from build123d import *


with BuildPart() as part:
    # Sketch2 → Revolve1 (revolve)
    with BuildSketch(Plane.XY, mode=Mode.PRIVATE) as revolve1_sk:
        with BuildLine():
            Line((-140, 65), (19.954223861, 65))
            add(Edge.make_bspline(
                [(19.954223861, 65), (21.016036949, 65.019364415), (23.155754142, 65.047133931), (27.308551501, 65.056367434), (32.353198871, 64.984650174), (38.152864496, 64.771098732), (45.567688357, 64.32486699), (54.255095035, 63.479775498), (63.813883484, 62.056181028), (72.567017756, 60.273903927), (83.242872896, 57.488773814), (94.867435167, 53.373767517), (106.518267243, 47.87450931), (116.322752818, 42.298539812), (124.736044428, 37.141710874), (132.197152427, 32.876448525), (139.118198638, 29.887038599), (146.009326462, 28.369530473), (153.724403185, 28.498164942), (163.163761497, 30.774524673), (172.93972339, 34.968320575), (182.118464779, 39.947020221), (189.735067248, 44.546297097), (198.139536323, 50.063346613), (205.847141634, 55.467762959), (212.465840749, 60.301248812), (217.661687494, 64.186041861), (222.197887983, 67.650369213), (225.939095655, 70.549100478), (227.873902956, 72.061946017), (228.830902799, 72.813469047)],
                knots=[0.000111982, 0.000111982, 0.000111982, 0.000111982, 0.007923607, 0.015735232, 0.031358482, 0.046981733, 0.062604983, 0.093851484, 0.125097984, 0.156344485, 0.187590985, 0.250083986, 0.312576987, 0.375069989, 0.43756299, 0.500055991, 0.562548992, 0.625041993, 0.687534994, 0.750027995, 0.812520997, 0.843767497, 0.875013998, 0.906260498, 0.937506999, 0.953130249, 0.968753499, 0.98437675, 0.992188375, 1, 1, 1, 1], degree=3))
            Line((228.830902799, 72.813469047), (231.918980433, 68.881068187))
            add(Edge.make_bspline(
                [(20.045394315, 60.000831274), (155.133832213, 62.464455683), (107.158700851, -29.09201306), (231.918980433, 68.881068187)],
                knots=[0.000111982, 0.000111982, 0.000111982, 0.000111982, 1, 1, 1, 1], degree=3))
            ThreePointArc((20.045394315, 60.000831274), (19.999810983, 60.000207823), (19.954223861, 60))
            Line((19.954223861, 60), (-140, 60))
            Line((-140, 60), (-140, 65))
        make_face()
    revolve(revolve1_sk.sketch.rotate(Axis((-140, 0, 0), (1, 0, 0)), 90), axis=Axis((-140, 0, 0), (1, 0, 0)))


solid = part.part
Verification items for the finished model (mm, model axes). Coordinates: 2 decimals unless noted, no trailing zeros. Loops run counter-clockwise (first coordinate to the right, second up) from the corner with the lowest first, then second, coordinate; pieces in that order, holes last. Notation, with made-up numbers: (55.25, 34.25) -> (90.25, 34.25) arc R27 ccw to (90.25, 56.25) -> close; hole circle Ø1 at (89, -18). An arc over 180 degrees is marked (long way). Answer as a JSON object with one key per item and string values. Group by question number.
Item 1: Mould release check, pull along Y, two halves, no side actions. Record for faces 1 (the cylindrical face through (-58.9, -19.52, 62)), 2 (the flat face through (-140, 57.5, -19)), 3 (the cylindrical face through (-61.14, -50.59, 32.26)): +Y half, -Y half, draft (parallel to the pull), parting line (faces both ways), or undercut.
Item 2: Sectioned sample at A-A on x = -98. Record the boundary of the cut face in (y, z), plus the area to 3 significant figures.
Item 3: Depth check by flat-ended pin: pin 1 (6 mm diameter, centred on x = 95, z = -7, fed in from -Y); pin 2 (1 mm diameter, centred on x = 13, z = -16, fed in from -Y); pin 3 (6 mm diameter, centred on x = 185.5, z = -11, fed in from -Y). Enter the tip coordinate at first touch or a pass-through.
Item 4: Scan lines: probe 1 along Y at (x, z) = (-78, 0); probe 2 along Y at (x, z) = (-48, -30); probe 3 along X at (y, z) = (-34, 18). Record each from-to range of solid material in increasing order.
Evaluation:
{
 "1": {"face 1": "parting line", "face 2": "draft", "face 3": "undercut"},
 "2": {"outline": "circle Ø130 at (0, 0); hole circle Ø120 at (0, 0)", "area": "1,960 mm²"},
 "3": {"pin 1": "stops at y = -53.87", "pin 2": "stops at y = -63.12", "pin 3": "stops at y = -42.58"},
 "4": {"probe 1": "y = -65 to -60, 60 to 65", "probe 2": "y = -57.66 to -51.96, 51.96 to 57.66", "probe 3": "x = 112.85 to 122.6, 179.36 to 189.31"}
}
